Check sheet for the modelled part. Datum: model origin and axes. Units: mm. Face numbers are marked on the shaded views. A direction names the side the tool comes from. Coordinates: 2 decimals unless noted, no trailing zeros. Loops run counter-clockwise (first coordinate to the right, second up) from the corner with the lowest first, then second, coordinate; pieces in that order, holes last. Notation, with made-up numbers: M 82,-23.75 L 88,-23.75 A14 ccw 88,-3.75 Z; hole C 73,39.25 d2. An arc over 180 degrees is marked long. Answer in a Markdown table with one row per item. Add a question column.
Autodesk Inventor part; units mm, degrees
ref_plane "YZ Plane" through (0, 0, 0) normal (1, 0, 0) x (0, 1, 0)
ref_plane "XZ Plane" through (0, 0, 0) normal (0, 1, 0) x (-1, 0, 0)
ref_plane "XY Plane" through (0, 0, 0) normal (0, 0, 1) x (1, 0, 0)
sketch "Sketch1" plane through (0, 0, 0) normal (0, 1, 0) x (-1, 0, 0)
  line L0 (125, 125) -> (-125, 125)
  line L1 (-125, 125) -> (-125, -125)
  line L2 (-125, -125) -> (125, -125)
  line L3 (125, -125) -> (125, 125)
  line L4 (125, 125) -> (-125, -125) construction
  line L5 (-125, 125) -> (125, -125) construction
  line L6 (-200, -200) -> (200, -200)
  line L7 (200, -200) -> (200, 200)
  line L8 (200, 200) -> (-200, 200)
  line L9 (-200, 200) -> (-200, -200)
  line L10 (-200, -200) -> (200, 200) construction
  line L11 (200, -200) -> (-200, 200) construction
  point P0 (0, 0)
  dimension "d0" = 250
  dimension "d1" = 250
  dimension "d2" = 400
  dimension "d3" = 400
extrude "Extrusion1" add sketch "Sketch1" along normal blind 75
sketch "Sketch2" plane through (0, 0, 0) normal (0, -1, 0) x (1, 0, 0)
  line L0 (-125, -125) -> (125, -125)
  line L1 (125, 125) -> (-125, 125)
  line L2 (-125, 125) -> (-125, -125)
  line L3 (-125, -125) -> (125, -125)
  line L4 (125, -125) -> (125, 125)
  line L5 (125, 125) -> (-125, -125) construction
  line L6 (-125, 125) -> (125, -125) construction
  point P0 (0, 0)
extrude "Extrusion2" add sketch "Sketch2" against normal blind 25
fillet "Fillet1" radius 50 4 edges at (200, 37.5, -200) (200, 37.5, 200) (-200, 37.5, -200) (-200, 37.5, 200)
sketch "Sketch3" plane through (0, 0, 0) normal (0, -1, 0) x (1, 0, 0)
  circle A0 centre (150, -150) radius 22.5
  arc A1 (150, -200) -> (200, -150) centre (150, -150) ccw
  circle A2 centre (-150, -150) radius 22.5
  circle A3 centre (-150, 150) radius 22.5
  circle A4 centre (150, 150) radius 22.5
  arc A5 (-200, -150) -> (-150, -200) centre (-150, -150) ccw
  arc A6 (-150, 200) -> (-200, 150) centre (-150, 150) ccw
  arc A7 (200, 150) -> (150, 200) centre (150, 150) ccw
  point P0 (0, 0)
  dimension "d9" = 45
  dimension "d10" = 45
  dimension "d11" = 45
  dimension "d12" = 45
extrude "Extrusion3" cut sketch "Sketch3" against normal blind 25
fillet "Fillet2" radius 125 4 edges at (-125, 50, -125) (-125, 50, 125) (125, 50, -125) (125, 50, 125)
sketch "Sketch4" plane through (0, 25, 0) normal (0, 1, 0) x (1, 0, 0)
  circle A0 centre (0, 0) radius 60
  dimension "d16" = 120
extrude "Extrusion4" cut sketch "Sketch4" against normal blind 10
properties part number "HANDBASE2"
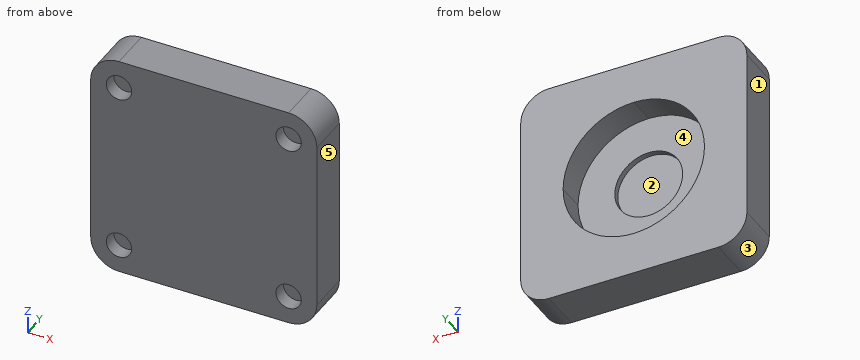
Q1. Access from +Z, -Z, +X, -X, +Y, -Y to the whole of each face (thin tool, end or side, straight path). Record for the marked faces 1 and 2.
Q2. Cross-section at D-D (x = 20). Record the cut outline in (y, z), plus the area to 3 significant figures.
Q3. Cross-section at A-A (y = 5). Record the cut outline in (x, z), plus the area to 3 significant figures.
Q4. Mould release check, pull along X, two halves, no side actions. Record for the marked faces 3, 4 and 5: released by +X, released by -X, zero draft, split by the parting line, or undercut.
Q5. Thickness scan on L1, parallel to Z at x = 150, y = 17; L2, parallel to X at y = 21.5, z = -39.5; L3, parallel to Z at x = 72.5, y = 54. Record the ranges inside material, lowest first.
Q6. Go/stop test with flat-tipped pins: pin 1 (3 mm diameter, centred on x = 152.5, y = 9.5, fed in from -Z); pin 2 (13.5 mm diameter, centred on x = -157.5, z = 144, fed in from -Y). Record where each tip stops, or that it passes through.
Q7. Cross-section at C-C (z = 140). Record the cut outline in (x, y), plus the area to 3 significant figures.
Answer key:
| question | item | result |
|---|---|---|
| 1 | face 1 | +Z, -Z, -X, +Y, -Y |
| 1 | face 2 | +Y |
| 2 | outline | M 0,-200 L 75,-200 L 75,-123.39 L 25,-123.39 L 25,-56.57 L 15,-56.57 L 15,56.57 L 25,56.57 L 25,123.39 L 75,123.39 L 75,200 L 0,200 Z |
| 2 | area | 16,500 mm^2 |
| 3 | outline | M -200,-150 A50 ccw -150,-200 L 150,-200 A50 ccw 200,-150 L 200,150 A50 ccw 150,200 L -150,200 A50 ccw -200,150 Z; hole C -150,-150 d45; hole C -150,150 d45; hole C 150,-150 d45; hole C 150,150 d45 |
| 3 | area | 151,000 mm^2 |
| 4 | face 3 | released by -X |
| 4 | face 4 | undercut |
| 4 | face 5 | released by +X |
| 5 | L1 | -200 to -172.5, -127.5 to 127.5, 172.5 to 200 |
| 5 | L2 | -200 to -45.16, 45.16 to 200 |
| 5 | L3 | -200 to -101.83, 101.83 to 200 |
| 6 | pin 1 | z = -199.99 |
| 6 | pin 2 | y = 25 |
| 7 | outline | M -200,0 L -170.16,0 L -170.16,25 L -129.84,25 L -129.84,0 L 129.84,0 L 129.84,25 L 170.16,25 L 170.16,0 L 200,0 L 200,75 L -200,75 Z |
| 7 | area | 28,000 mm^2 |
